```python
from build123d import *

# Parameters (mm, degrees)
SKETCH1_W                    = 35
SKETCH1_H                    = 35
SKETCH1_R                    = 4.05
SKETCH1_R_2                  = 1.6
BOSS_EXTRUDE1_DEPTH          = 12
FILLET1_R                    = 5
SKETCH5_R                    = 3.2
CUT_EXTRUDE1_DEPTH           = 1
CUT_EXTRUDE1_DRAFT           = -60
CUT_EXTRUDE1_PROFILE_2_DEPTH = 1
CUT_EXTRUDE1_PROFILE_2_DRAFT = -60
CUT_EXTRUDE1_PROFILE_3_DEPTH = 1
CUT_EXTRUDE1_PROFILE_3_DRAFT = -60
CUT_EXTRUDE1_PROFILE_4_DEPTH = 1
CUT_EXTRUDE1_PROFILE_4_DRAFT = -60
CUT_EXTRUDE2_DEPTH           = 7


with BuildPart() as part:
    # Sketch1 → Boss-Extrude1 (new body)
    with BuildSketch(Plane.XY):
        Rectangle(SKETCH1_W, SKETCH1_H)
        Circle(SKETCH1_R, mode=Mode.SUBTRACT)
        with Locations((-9.25, 8.75)):
            Circle(SKETCH1_R_2, mode=Mode.SUBTRACT)
        with Locations((9.25, 8.75)):
            Circle(SKETCH1_R_2, mode=Mode.SUBTRACT)
        with Locations((-9.25, -8.75)):
            Circle(SKETCH1_R_2, mode=Mode.SUBTRACT)
        with Locations((9.25, -8.75)):
            Circle(SKETCH1_R_2, mode=Mode.SUBTRACT)
    extrude(amount=BOSS_EXTRUDE1_DEPTH)

    # Fillet1
    fillet1_edges = [part.edges().sort_by_distance(p)[0] for p in [
        (-17.5, -17.5, 6),
        (-17.5, 17.5, 6),
        (17.5, 17.5, 6),
        (17.5, -17.5, 6),
    ]]
    fillet(fillet1_edges, radius=FILLET1_R)


with BuildPart() as cut_extrude1_tool:
    # Sketch5 → Cut-Extrude1 (with draft: the straight prism first)
    with BuildSketch(Plane.XY.offset(12)):
        with Locations((-9.25, 8.75)):
            Circle(SKETCH5_R)
    extrude(amount=-CUT_EXTRUDE1_DEPTH)
    # Cut-Extrude1: the draft: its side faces are tilted about the plane it starts from
    cut_extrude1_sides = [cut_extrude1_tool.faces().sort_by_distance(p)[0] for p in [
        (-12.45, 8.75, 11.5),
    ]]
    draft(cut_extrude1_sides, Plane.XY.offset(12), CUT_EXTRUDE1_DRAFT)


with BuildPart() as part_1:
    add(part.part)

    # Cut-Extrude1: cut by cut_extrude1_tool
    add(cut_extrude1_tool.part, mode=Mode.SUBTRACT)


with BuildPart() as cut_extrude1_profile_2_tool:
    # Sketch5 → Cut-Extrude1 profile 2 (with draft: the straight prism first)
    with BuildSketch(Plane.XY.offset(12)):
        with Locations((9.25, 8.75)):
            Circle(SKETCH5_R)
    extrude(amount=-CUT_EXTRUDE1_PROFILE_2_DEPTH)
    # Cut-Extrude1 profile 2: the draft: its side faces are tilted about the plane it starts from
    cut_extrude1_profile_2_sides = [cut_extrude1_profile_2_tool.faces().sort_by_distance(p)[0] for p in [
        (6.05, 8.75, 11.5),
    ]]
    draft(cut_extrude1_profile_2_sides, Plane.XY.offset(12), CUT_EXTRUDE1_PROFILE_2_DRAFT)


with BuildPart() as part_2:
    add(part_1.part)

    # Cut-Extrude1 profile 2: cut by cut_extrude1_profile_2_tool
    add(cut_extrude1_profile_2_tool.part, mode=Mode.SUBTRACT)


with BuildPart() as cut_extrude1_profile_3_tool:
    # Sketch5 → Cut-Extrude1 profile 3 (with draft: the straight prism first)
    with BuildSketch(Plane.XY.offset(12)):
        with Locations((-9.25, -8.75)):
            Circle(SKETCH5_R)
    extrude(amount=-CUT_EXTRUDE1_PROFILE_3_DEPTH)
    # Cut-Extrude1 profile 3: the draft: its side faces are tilted about the plane it starts from
    cut_extrude1_profile_3_sides = [cut_extrude1_profile_3_tool.faces().sort_by_distance(p)[0] for p in [
        (-12.45, -8.75, 11.5),
    ]]
    draft(cut_extrude1_profile_3_sides, Plane.XY.offset(12), CUT_EXTRUDE1_PROFILE_3_DRAFT)


with BuildPart() as part_3:
    add(part_2.part)

    # Cut-Extrude1 profile 3: cut by cut_extrude1_profile_3_tool
    add(cut_extrude1_profile_3_tool.part, mode=Mode.SUBTRACT)


with BuildPart() as cut_extrude1_profile_4_tool:
    # Sketch5 → Cut-Extrude1 profile 4 (with draft: the straight prism first)
    with BuildSketch(Plane.XY.offset(12)):
        with Locations((9.25, -8.75)):
            Circle(SKETCH5_R)
    extrude(amount=-CUT_EXTRUDE1_PROFILE_4_DEPTH)
    # Cut-Extrude1 profile 4: the draft: its side faces are tilted about the plane it starts from
    cut_extrude1_profile_4_sides = [cut_extrude1_profile_4_tool.faces().sort_by_distance(p)[0] for p in [
        (6.05, -8.75, 11.5),
    ]]
    draft(cut_extrude1_profile_4_sides, Plane.XY.offset(12), CUT_EXTRUDE1_PROFILE_4_DRAFT)


with BuildPart() as part_4:
    add(part_3.part)

    # Cut-Extrude1 profile 4: cut by cut_extrude1_profile_4_tool
    add(cut_extrude1_profile_4_tool.part, mode=Mode.SUBTRACT)

    # Sketch6 → Cut-Extrude2 (cut)
    with BuildSketch(Plane(origin=(0, 0, 0), x_dir=(-1, 0, 0), z_dir=(0, 0, -1))):
        Polygon((6.538491799, 3.775), (0, 7.55), (-6.538491799, 3.775), (-6.538491799, -3.775), (0, -7.55), (6.538491799, -3.775), align=None)
    extrude(amount=-CUT_EXTRUDE2_DEPTH, mode=Mode.SUBTRACT)


solid = part_4.part
```
The listing builds one solid part. Answer for the finished solid, in the listing's coordinates (mm). A direction names the side the tool comes from. Give positions to 0.01 mm unless a question says otherwise; leave off trailing zeros. Order: outer loops, then holes, each group sorted by start corner. A loop starts at its lowest first (then second) coordinate and runs counter-clockwise, first axis right, second up.
Item 1: Given pin 1 Ø3 at (x, y) = (9.25, 8.75) entering from -Z; pin 2 Ø5 at (x, y) = (-9.25, 8.75) entering from +Z; pin 3 Ø10.5 at (x, y) = (0, 0) entering from -Z; pin 4 Ø4 at (x, y) = (-9.25, -8.75) entering from +Z, each flat-ended and moving along its own axis, determine where each tip first touches the part or whether it passes through.
From the geometry:
pin 1: passes through
pin 2: stops at z = 11.6
pin 3: stops at z = 7
pin 4: stops at z = 11.31
Item 2: The part is cut by section D-D, the plane y = 0. Give the vertices of the cut face in (x, z), and give its area (3 significant figures).
From the geometry:
outline: (-17.5, 0) - (-6.54, 0) - (-6.54, 7) - (-4.05, 7) - (-4.05, 12) - (-17.5, 12) - close; (4.05, 7) - (6.54, 7) - (6.54, 0) - (17.5, 0) - (17.5, 12) - (4.05, 12) - close
area: 288 mm2
Item 3: The part is cut by section B-B, the plane z = 9.75. Give the vertices of the cut face in (x, y), and give its area (3 significant figures).
From the geometry:
outline: (-17.5, -12.5) arc R5 ccw to (-12.5, -17.5) - (12.5, -17.5) arc R5 ccw to (17.5, -12.5) - (17.5, 12.5) arc R5 ccw to (12.5, 17.5) - (-12.5, 17.5) arc R5 ccw to (-17.5, 12.5) - close; hole circle Ø3.2 at (-9.25, -8.75); hole circle Ø3.2 at (-9.25, 8.75); hole circle Ø8.1 at (0, 0); hole circle Ø3.2 at (9.25, -8.75); hole circle Ø3.2 at (9.25, 8.75)
area: 1,120 mm2
Item 4: For a pull along Y with two mould halves and no side action, classify faces 1 (the face through (-16.07, 16, 6.08)), 2 (the face through (-10.85, -8.68, 5.46)), 3 (the face through (8, 0, 0)) as pulls with the +Y half, pulls with the -Y half, needs draft (parallel to the pull), parting line crosses it, or undercut.
From the geometry:
face 1: pulls with the +Y half
face 2: undercut
face 3: needs draft
Item 5: The part is cut by section A-A, the plane y = 8.75. Give the vertices of the cut face in (x, z).
From the geometry:
outline: (-17.5, 0) - (-10.85, 0) - (-10.85, 11.08) - (-12.45, 12) - (-17.5, 12) - close; (-7.65, 0) - (7.65, 0) - (7.65, 11.08) - (6.05, 12) - (-6.05, 12) - (-7.65, 11.08) - close; (10.85, 0) - (17.5, 0) - (17.5, 12) - (12.45, 12) - (10.85, 11.08) - close
Item 6: The part is cut by section C-C, the plane x = 9.25. Give the vertices of the cut face in (y, z).
From the geometry:
outline: (-17.5, 0) - (-10.35, 0) - (-10.35, 11.08) - (-11.95, 12) - (-17.5, 12) - close; (-7.15, 0) - (7.15, 0) - (7.15, 11.08) - (5.55, 12) - (-5.55, 12) - (-7.15, 11.08) - close; (10.35, 0) - (17.5, 0) - (17.5, 12) - (11.95, 12) - (10.35, 11.08) - close
Item 7: Find the intervals of material crossed by probe 1 along X at (y, z) = (8.75, 3.5); probe 2 along Y at (x, z) = (-9.25, 6.75); probe 3 along X at (y, z) = (-8, 0.5), in increasing order.
From the geometry:
probe 1: x = -17.5 to -10.85, -7.65 to 7.65, 10.85 to 17.5
probe 2: y = -17.5 to -10.35, -7.15 to 7.15, 10.35 to 17.5
probe 3: x = -17.5 to -10.66, -7.84 to 7.84, 10.66 to 17.5
Item 8: Which of the six approach directions +Z, -Z, +X, -X, +Y, -Y give full straight-line access (tool end or side, diameter ignored) to faces 4 (the face through (-6.538, 0, 3)), 5 (the face through (0, 17.5, 6))?
From the geometry:
face 4: -Z
face 5: +Z, -Z, +X, -X, +Y
